For this review, take the finished solid that the model builds, in its own axes (mm). Give positions to 0.01 mm unless a question says otherwise; leave off trailing zeros. Write each loop counter-clockwise with the first axis right and the second up, starting at its lowest first coordinate (ties: lowest second). Pieces come first, ordered by that corner, then holes.
1) We need section B-B on z = 2.25. Give the number of separate pieces and of enclosed holes in the cut face, and give its area (3 significant figures).
2) For P1, Ø6.5, axis at y = 1, z = 8, coming from the +X side; P2, Ø5.5, axis at x = 87, y = 0, coming from the -Z side, all flat-tipped, find the tip position at first contact; note any pin that passes through.
3) We need section D-D on x = 32. Give the boundary of the cut face in (y, z).
4) We need section A-A on x = 69.6. Give the boundary of the cut face in (y, z).
5) Wall thickness on line 1 along X through (y, z) = (9, 8); line 2 along X through (y, z) = (8.5, 8.5); line 3 along Z through (x, y) = (-26, -4): over which ranges is each line inside the solid? List them lowest first.
from build123d import *

# Parameters (mm, degrees)
F0_W           = 174
F0_H           = 20
F0_R           = 4.6
F1_DEPTH       = 4
F2_W           = 14
F2_H           = 20
F3_DEPTH       = 7.5
F5_D           = 4.6
F5_CBORE_D     = 7.5
F5_CBORE_DEPTH = 8
F6_R           = 6.99999
F7_DEPTH       = 7.5
F8_W           = 3
F8_H           = 6.5
F9_DEPTH       = 25
F10_W          = 4
F10_H          = 7.5
F11_DEPTH      = 7
F12_R          = 2.3
F13_DEPTH      = 10


# Not quite as in the source:
# - a fillet or chamfer is up to 0.001 mm smaller than in the source, because OpenCascade refuses the exact size


with BuildPart() as f1:
    # F0 (on Top) → F1 (new body)
    with BuildSketch(Plane.XY):
        with Locations((52.2, 0)):
            Rectangle(F0_W, F0_H)
        Circle(F0_R, mode=Mode.SUBTRACT)
        with Locations((34.8, 0)):
            Circle(F0_R, mode=Mode.SUBTRACT)
        with Locations((69.6, 0)):
            Circle(F0_R, mode=Mode.SUBTRACT)
        with Locations((104.4, 0)):
            Circle(F0_R, mode=Mode.SUBTRACT)
    extrude(amount=F1_DEPTH)

    # F2 (on face) → F3 (join)
    with BuildSketch(Plane.XY.offset(4)):
        with Locations((-17.4, 0)):
            Rectangle(F2_W, F2_H)
        with Locations((17.4, 0)):
            Rectangle(F2_W, F2_H)
        with Locations((52.2, 0)):
            Rectangle(F2_W, F2_H)
        with Locations((87, 0)):
            Rectangle(F2_W, F2_H)
        with Locations((121.8, 0)):
            Rectangle(F2_W, F2_H)
    extrude(amount=F3_DEPTH)

    # F5 (through all)
    with Locations(Plane(origin=(0, 0, 0), x_dir=(1, 0, 0), z_dir=(0, 0, -1))):
        with Locations((-17.4, 0), (17.4, 0), (52.2, 0), (87, 0), (121.8, 0)):
            CounterBoreHole(F5_D / 2, F5_CBORE_D / 2, F5_CBORE_DEPTH)

    # F6 (radius 7 in the source; OpenCascade refuses exactly that, so slightly less here)
    f6_edges = [f1.edges().sort_by_distance(p)[0] for p in [
        (-10.4, 10, 7.75),
        (10.4, 10, 7.75),
        (24.4, 10, 7.75),
        (45.2, 10, 7.75),
        (59.2, 10, 7.75),
        (80, 10, 7.75),
        (94, 10, 7.75),
        (128.8, 10, 7.75),
        (114.8, 10, 7.75),
        (-24.4, 10, 7.75),
        (-24.4, -10, 7.75),
        (-10.4, -10, 7.75),
        (10.4, -10, 7.75),
        (24.4, -10, 7.75),
        (45.2, -10, 7.75),
        (59.2, -10, 7.75),
        (80, -10, 7.75),
        (94, -10, 7.75),
        (114.8, -10, 7.75),
        (128.8, -10, 7.75),
    ]]
    fillet(f6_edges, radius=F6_R)

    # F7 (add): a face of the model
    f7_faces = [f1.faces().sort_by_distance(p)[0] for p in [
        (-28.9789302808, 0, 4),
    ]]
    extrude(f7_faces, amount=F7_DEPTH)

    # F8 (on face) → F9 (cut)
    with BuildSketch(Plane(origin=(0, 10, 0), x_dir=(-1, 0, 0), z_dir=(0, 1, 0))):
        with Locations((26.3, 7.25)):
            Rectangle(F8_W, F8_H)
    extrude(amount=-F9_DEPTH, mode=Mode.SUBTRACT)

    # F10 (on face) → F11 (cut)
    with BuildSketch(Plane.XY.offset(11.5)):
        with Locations((-28.5152019933, 0)):
            Rectangle(F10_W, F10_H)
    extrude(amount=-F11_DEPTH, mode=Mode.SUBTRACT)

    # F12 (on face) → F13 (cut)
    with BuildSketch(Plane(origin=(-34.8, 0, 0), x_dir=(0, -1, 0), z_dir=(-1, 0, 0))):
        with Locations((0, 7.5)):
            Circle(F12_R)
    extrude(amount=-F13_DEPTH, mode=Mode.SUBTRACT)


solid = f1.part
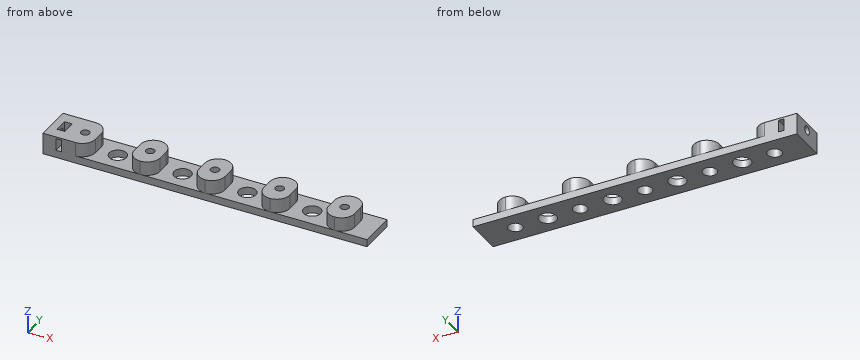
Results list:
1. separate pieces: 1
1. enclosed holes: 9
1. area: 2,990 mm2
2. P1: stops at x = 128.8
2. P2: stops at z = 8
3. outline: (-10, 0) - (-3.65, 0) - (-3.65, 4) - (-10, 4) - close; (3.65, 0) - (10, 0) - (10, 4) - (3.65, 4) - close
4. outline: (-10, 0) - (-4.6, 0) - (-4.6, 4) - (-10, 4) - close; (4.6, 0) - (10, 0) - (10, 4) - (4.6, 4) - close
5. line 1: x = -34.8 to -27.8, -24.8 to -13.79, 13.79 to 21.01, 48.59 to 55.81, 83.39 to 90.61, 118.19 to 125.41
5. line 2: x = -34.8 to -27.8, -24.8 to -13.07, 13.07 to 21.73, 47.87 to 56.53, 82.67 to 91.33, 117.47 to 126.13
5. line 3: z = 0 to 4, 10.5 to 11.5
